from build123d import *

# Parameters (mm, degrees)
SKETCH_1_R          = 3
EXTRUDE_1_DEPTH     = 14
SKETCH_2_R          = 7
SKETCH_2_R_2        = 4
EXTRUDE_2_DEPTH     = 8
CUT_EXTRUDE_START   = -4
SKETCH_2_2_R        = 4
CUT_EXTRUDE_1_DEPTH = 4


with BuildPart() as part:
    # Sketch 1 → Extrude 1 (new body)
    with BuildSketch(Plane(origin=(0, 0, 0), x_dir=(1, 0, 0), z_dir=(0, 1, 0))):
        with BuildLine():
            Line((-5, 7.5), (5, 7.5))
            ThreePointArc((5, 7.5), (12.5, 0), (5, -7.5))
            Line((5, -7.5), (-5, -7.5))
            Line((-5, -7.5), (-5, 7.5))
        make_face()
        with Locations(Location((5, 0, 0), (0, 0, 270))):
            Circle(SKETCH_1_R, mode=Mode.SUBTRACT)
    extrude(amount=EXTRUDE_1_DEPTH)

    # Sketch 2 → Extrude 2 (add)
    with BuildSketch(Plane.ZY.offset(5)):
        with Locations(Location((0, 7, 0), (0, 0, 270))):
            Circle(SKETCH_2_R)
        with Locations((0, 7)):
            Circle(SKETCH_2_R_2, mode=Mode.SUBTRACT)
    extrude(amount=EXTRUDE_2_DEPTH)

    # Sketch 2_2 → Cut-Extrude 1 (cut)
    with BuildSketch(Plane.ZY.offset(5).offset(CUT_EXTRUDE_START)):
        with Locations((0, 7)):
            Circle(SKETCH_2_2_R)
    extrude(amount=CUT_EXTRUDE_1_DEPTH, mode=Mode.SUBTRACT)


solid = part.part
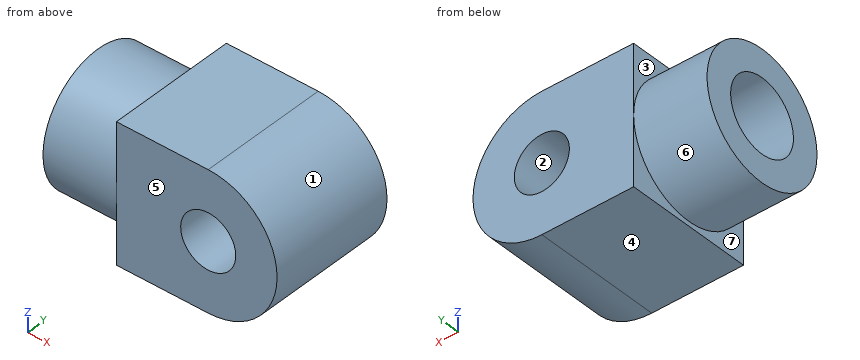
Build history of the part. All positions in model axes, mm. Face numbers are marked on the shaded views. A direction names the side the tool comes from. Round coordinates to 2 decimals unless told otherwise and drop trailing zeros. Loops run counter-clockwise (first coordinate to the right, second up) from the corner with the lowest first, then second, coordinate; pieces in that order, holes last. Notation, with made-up numbers: (33, -9.75) -> (47, -9.75) arc R15 ccw to (47, 15.25) -> close; hole circle Ø5 at (-1.75, 30). An arc over 180 degrees is marked (long way). Answer in a Markdown table with one row per item.
Item 1: Saw through at C-C (z = 2.5). Write the cut outline in (x, y), and give its area (3 significant figures).
Answers below:
| item | result |
|---|---|
| outline | (-13, 0.46) -> (-5, 0.46) -> (-5, 0) -> (3.34, 0) -> (3.34, 14) -> (-5, 14) -> (-5, 13.54) -> (-13, 13.54) -> (-13, 10.12) -> (-1, 10.12) -> (-1, 3.88) -> (-13, 3.88) -> close; (6.66, 0) -> (12.07, 0) -> (12.07, 14) -> (6.66, 14) -> close |
| area | 222 mm² |
Item 2: Saw through at A-A (x = 4). Write the cut outline in (y, z).
Answers below:
| item | result |
|---|---|
| outline | (0, -7.5) -> (14, -7.5) -> (14, -2.83) -> (0, -2.83) -> close; (0, 2.83) -> (14, 2.83) -> (14, 7.5) -> (0, 7.5) -> close |
Item 3: Pin check, flat tips, straight feed: pin 1 (4 mm diameter, centred on y = 6.5, z = -0.5, fed in from -X); pin 2 (1.5 mm diameter, centred on x = -10, y = 8, fed in from -Z); pin 3 (1.5 mm diameter, centred on x = -7.5, y = 9, fed in from +Z). Stop position of each tip, or through.
Answers below:
| item | result |
|---|---|
| pin 1 | stops at x = -1 |
| pin 2 | stops at z = -7 |
| pin 3 | stops at z = 6.89 |
Item 4: Which spindle directions (+Z, -Z, +X, -X, +Y, -Y) get a long thin tool onto all of the face, cutting with end or side? Do the marked faces 5, 6 and 7. Say none if no direction does.
Answers below:
| item | result |
|---|---|
| face 5 | +Z, -Z, +X, -X, -Y |
| face 6 | -X |
| face 7 | -Z, -X |
Item 5: Saw through at B-B (y = 7). Write the cut outline in (x, z), and give its area (3 significant figures).
Answers below:
| item | result |
|---|---|
| outline | (-13, -7) -> (-5, -7) -> (-5, -7.5) -> (5, -7.5) arc R7.5 ccw to (5, 7.5) -> (-5, 7.5) -> (-5, 7) -> (-13, 7) -> (-13, 4) -> (-1, 4) -> (-1, -4) -> (-13, -4) -> close; hole circle Ø6 at (5, 0) |
| area | 226 mm² |
Item 6: Saw through at D-D (x = -8.5). Write the cut outline in (y, z).
Answers below:
| item | result |
|---|---|
| outline | circle Ø14 at (7, 0); hole circle Ø8 at (7, 0) |
Item 7: Mould opens along Z. For the marked faces 1, 2, 3 and 4 say: +Z half, -Z half, draft (parallel to the pull), parting line (faces both ways), or undercut.
Answers below:
| item | result |
|---|---|
| face 1 | parting line |
| face 2 | undercut |
| face 3 | draft |
| face 4 | -Z half |
Item 8: Drill centre lines: L1, parallel to X at y = 11.25, z = 0; L2, parallel to X at y = 6.25, z = 0; L3, parallel to Y at x = -5.75, z = 3.5. Where is each one in solid material? Low to high. Write a range as [from, to].
Answers below:
| item | result |
|---|---|
| L1 | x = [-13, 2], [8, 12.5] |
| L2 | x = [-1, 2], [8, 12.5] |
| L3 | y = [0.94, 5.06], [8.94, 13.06] |
